Autodesk Inventor part; units mm, degrees
ref_plane "YZ Plane" through (0, 0, 0) normal (1, 0, 0) x (0, 1, 0)
ref_plane "XZ Plane" through (0, 0, 0) normal (0, 1, 0) x (-1, 0, 0)
ref_plane "XY Plane" through (0, 0, 0) normal (0, 0, 1) x (1, 0, 0)
sketch "Skizze1" plane through (0, 0, 0) normal (0, 1, 0) x (-1, 0, 0)
  line L0 (0, 0) -> (14, 0)
  line L1 (14, 0) -> (14, -10)
  line L2 (14, -10) -> (5, -10)
  line L3 (5, -10) -> (5, -20)
  line L4 (5, -20) -> (0, -20)
  line L5 (0, -20) -> (0, 0)
  point P0 (9.5, -10)
  dimension "d0" = 10
  dimension "d1" = 10
  dimension "d2" = 10
  dimension "d3" = 28
revolve "Umdrehung1" add sketch "Skizze1" angle 360 about axis through (0, 0, -20) along (0, 0, 1)
sketch "Skizze2" plane through (0, 0, 0) normal (0, 0, 1) x (1, 0, 0)
  circle A0 centre (0, 0) radius 14
  point P0 (0, 0)
hole "Bohrung1" at (0, 0, 0) direction (0, 0, -1) diameter 6.5 depth 20
sketch "Skizze4" plane through (0, 0, 0) normal (0, 1, 0) x (-1, 0, 0)
  line L0 (-3.25, 0) -> (3.25, 0)
  point P0 (0, 0)
  point P1 (0, -5)
  dimension "d12" = 5
hole "Bohrung2" at (0, 0, -5) direction (0, -1, 0) diameter 3.242 end through all
mirror "Spiegeln1" about plane through (0, 0, 0) normal (0, 1, 0) of "Bohrung2"
chamfer "Fasen1" distance 1 angle 45 1 edges at (14, 0, -10)
properties part number "30" material "Kupfer"
Design review of the part built by this model. Coordinates are the model's own, in mm. A direction names the side the tool comes from. Coordinates: 2 decimals unless noted, no trailing zeros. Order: outer loops, then holes, each group sorted by start corner. A loop starts at its lowest first (then second) coordinate and runs counter-clockwise, first axis right, second up.
Item 1: Take a section at B-B, the plane x = 0. Write out the cut boundary in (y, z), then the cut area to 3 significant figures.
Item 2: Take a section at C-C, the plane z = -5.25. Write out the cut boundary in (x, y), then the cut area to 3 significant figures.
Item 3: For pin 1 Ø1 at (x, z) = (11, -5.5) entering from +Y; pin 2 Ø3 at (x, z) = (0.5, -10) entering from +Y; pin 3 Ø4 at (x, z) = (4.5, -7) entering from -Y (3 decimals); pin 4 Ø8 at (x, y) = (-9.5, -2) entering from -Z, all flat-tipped, find the tip position at first contact; note any pin that passes through.
Item 4: Take a section at A-A, the plane y = 0. Write out the cut boundary in (x, z), then the cut area to 3 significant figures.
Item 5: Take a section at D-D, the plane z = -12.25. Write out the cut boundary in (x, y).
Item 6: For faces 1 (the cylindrical face through (-0.07, -8.49, -6.62)), 2 (the flat face through (-6, 0, -10)), list the 3-axis set-ups (+Z, -Z, +X, -X, +Y, -Y) from which the entire face can be reached by the end or side of a thin tool; tool diameter is ignored.
Item 7: The part is to be moulded in two halves that separate along X. For faces 3 (the cylindrical face through (-12.932, -5.362, -4.563)), 4 (the cylindrical face through (-0.98, -3.1, -10.14)), 5 (the flat face through (-3, 3, 0)), say which applies: pulls with the +X half, pulls with the -X half, needs draft (parallel to the pull), parting line crosses it, or undercut.
Item 8: For line 1 (Z direction, x = 0, y = -10.25); line 2 (Y direction, x = 0, z = -15.5); line 3 (Z direction, x = 10.5, y = 1.75), list the stretches that pass through material, from the lowest coordinate up.
The answers:
1. outline: (-14, -9) - (-13, -10) - (-5, -10) - (-5, -20) - (-3.25, -20) - (-3.25, -6.62) - (-14, -6.62) - close; (-14, -3.38) - (-3.25, -3.38) - (-3.25, 0) - (-14, 0) - close; (3.25, -20) - (5, -20) - (5, -10) - (13, -10) - (14, -9) - (14, -6.62) - (3.25, -6.62) - close; (3.25, -3.38) - (14, -3.38) - (14, 0) - (3.25, 0) - close
1. area: 179 mm2
2. outline: (-1.6, -13.91) - (-1.6, -2.83) arc R3.25 cw to (-1.6, 2.83) - (-1.6, 13.91) arc R14 ccw to start; (1.6, -13.91) arc R14 ccw to (1.6, 13.91) - (1.6, 2.83) arc R3.25 cw to (1.6, -2.83) - close
2. area: 513 mm2
3. pin 1: stops at y = 9.26
3. pin 2: stops at y = 14
3. pin 3: stops at y = -13.775
3. pin 4: stops at z = -10
4. outline: (-14, -9) - (-13, -10) - (-5, -10) - (-5, -20) - (-3.25, -20) - (-3.25, 0) - (-14, 0) - close; (3.25, -20) - (5, -20) - (5, -10) - (13, -10) - (14, -9) - (14, 0) - (3.25, 0) - close
4. area: 249 mm2
5. outline: circle Ø10 at (0, 0); hole circle Ø6.5 at (0, 0)
6. face 1: +Y, -Y
6. face 2: -Z
7. face 3: parting line crosses it
7. face 4: undercut
7. face 5: needs draft
8. line 1: z = -10 to -6.62, -3.38 to 0
8. line 2: y = -5 to -3.25, 3.25 to 5
8. line 3: z = -10 to 0
